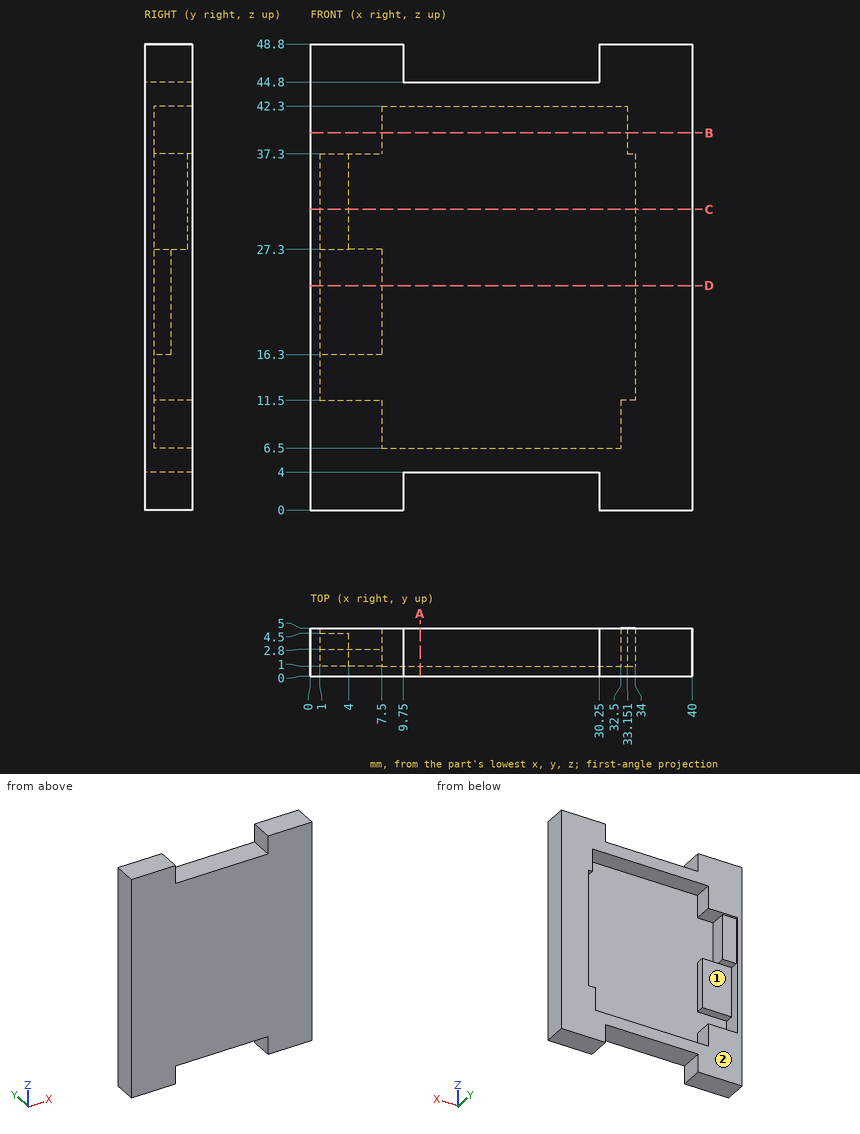
Check sheet for the drawn part. Datum: minimum x, y, z corner. Units: mm. Round coordinates to 2 decimals unless told otherwise and drop trailing zeros. Write each loop counter-clockwise with the first axis right and the second up, starting at its lowest first coordinate (ties: lowest second). Pieces come first, ordered by that corner, then holes. Notation, with made-up numbers: (23.5, 33) -> (30.5, 33) arc R38 cw to (30.5, 71) -> close; hole circle Ø6 at (72, 6). An arc over 180 degrees is marked (long way). One line per item, written item: value. Start each with the question number.
(1) Cross-section at B-B, the plane z = 39.5. Record the cut outline in (x, y).
(2) Cross-section at A-A, the plane x = 11.5. Record the cut outline in (y, z), and give its area (3 significant figures).
(3) Go/stop test with flat-tipped pins: pin 1 Ø6 at (x, z) = (29, 32.5) entering from +Y; pin 2 Ø3 at (x, z) = (3.5, 21.5) entering from +Y; pin 3 Ø2.5 at (x, y) = (15.5, 3.5) entering from +Z. Record where each tip stops, or that it passes through.
(4) Draft check along Z on the marked faces 1 and 2. Enter one of: +Z half, -Z half, draft (parallel to the pull), parting line (faces both ways), or undercut.
(5) Cross-section at C-C, the plane z = 31.5. Record the cut outline in (x, y).
(6) Scan lines: line 1 (X direction, y = 3.75, z = 27.5); line 2 (X direction, y = 2.45, z = 45); line 3 (Z direction, x = 16, y = 4.1). Record each from-to range of solid material in increasing order. Write a range as [from, to].
(7) Cross-section at D-D, the plane z = 23.5. Record the cut outline in (x, y), and give its area (3 significant figures).
Answer:
1. outline: (0, 0) -> (40, 0) -> (40, 5) -> (33.15, 5) -> (33.15, 1) -> (7.5, 1) -> (7.5, 5) -> (0, 5) -> close
2. outline: (0, 4) -> (5, 4) -> (5, 6.5) -> (1, 6.5) -> (1, 42.3) -> (5, 42.3) -> (5, 44.8) -> (0, 44.8) -> close
2. area: 60.8 mm²
3. pin 1: y = 1
3. pin 2: y = 2.8
3. pin 3: z = 44.8
4. face 1: undercut
4. face 2: draft
5. outline: (0, 0) -> (40, 0) -> (40, 5) -> (34, 5) -> (34, 1) -> (4, 1) -> (4, 4.5) -> (1, 4.5) -> (1, 5) -> (0, 5) -> close
6. line 1: [0, 4], [34, 40]
6. line 2: [0, 9.75], [30.25, 40]
6. line 3: [4, 6.5], [42.3, 44.8]
7. outline: (0, 0) -> (40, 0) -> (40, 5) -> (34, 5) -> (34, 1) -> (7.5, 1) -> (7.5, 2.8) -> (1, 2.8) -> (1, 5) -> (0, 5) -> close
7. area: 79.7 mm²
